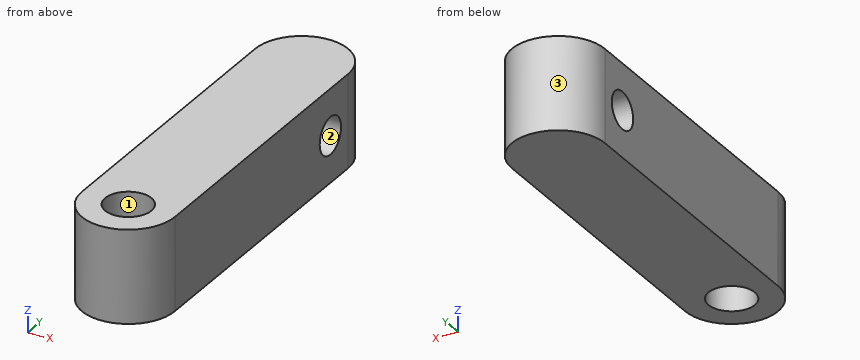
from build123d import *

# Parameters (mm, degrees)
SKETCH2_R           = 5
BOSS_EXTRUDE1_DEPTH = 20
SKETCH4_R           = 4
CUT_EXTRUDE1_DEPTH  = 55


with BuildPart() as part:
    # Sketch2 → Boss-Extrude1 (new body)
    with BuildSketch(Plane.XY):
        with BuildLine():
            Line((-10, 0), (-10, 65))
            ThreePointArc((-10, 65), (0, 75), (10, 65))
            Line((10, 65), (10, 0))
            ThreePointArc((10, 0), (0, -10), (-10, 0))
        make_face()
        Circle(SKETCH2_R, mode=Mode.SUBTRACT)
    extrude(amount=BOSS_EXTRUDE1_DEPTH)

    # Sketch4 → Cut-Extrude1 (cut)
    with BuildSketch(Plane(origin=(10, 0, 0), x_dir=(0, 0, -1), z_dir=(1, 0, 0))):
        with Locations((-10, 58.36)):
            Circle(SKETCH4_R)
    extrude(amount=-CUT_EXTRUDE1_DEPTH, mode=Mode.SUBTRACT)


solid = part.part
Verification items for the finished model (mm, model axes). Face numbers are marked on the shaded views. Round coordinates to 2 decimals unless told otherwise and drop trailing zeros. Loops run counter-clockwise (first coordinate to the right, second up) from the corner with the lowest first, then second, coordinate; pieces in that order, holes last. Notation, with made-up numbers: (17, 50.5) - (65, 50.5) arc R11 ccw to (65, 69.5) - close; hole circle Ø4 at (-38, 76). An arc over 180 degrees is marked (long way). Use a Markdown table: item, result. Add a question column.
1. Section check A-A, the plane z = 10. Record the boundary of the cut face in (x, y).
2. Section check D-D, the plane x = 7.5. Record the boundary of the cut face in (y, z), plus the area to 3 significant figures.
3. Thickness scan on probe 1 along Y at (x, z) = (0, 10); probe 2 along Y at (x, z) = (4.25, 8.75); probe 3 along Y at (x, z) = (-2.75, 19.25). Record the ranges inside material, lowest first. Write a range as [from, to].
4. Gauge pin test, flat ends, axial feed: pin 1 (3 mm diameter, centred on x = 7, z = 3, fed in from +Y); pin 2 (1 mm diameter, centred on x = 7.5, z = 7, fed in from +Y); pin 3 (1.5 mm diameter, centred on x = 5, z = 17, fed in from +Y). Record the tip position at first contact, or that the pin passes through.
5. Section check C-C, the plane y = 58.36. Record the boundary of the cut face in (x, z).
6. Release check for a two-part mould opening along X. For the marked faces 1, 2 and 3 record: released by +X, released by -X, zero draft, split by the parting line, or undercut.
7. Section check B-B, the plane x = -1. Record the boundary of the cut face in (y, z).
Checks:
| question | item | result |
|---|---|---|
| 1 | outline | (-10, 0) arc R10 ccw to (10, 0) - (10, 54.36) - (-10, 54.36) - close; (-10, 62.36) - (10, 62.36) - (10, 65) arc R10 ccw to (-10, 65) - close; hole circle Ø10 at (0, 0) |
| 2 | outline | (-6.61, 0) - (71.61, 0) - (71.61, 20) - (-6.61, 20) - close; hole circle Ø8 at (58.36, 10) |
| 2 | area | 1,510 mm^2 |
| 3 | probe 1 | y = [-10, -5], [5, 54.36], [62.36, 75] |
| 3 | probe 2 | y = [-9.05, -2.63], [2.63, 54.56], [62.16, 74.05] |
| 3 | probe 3 | y = [-9.61, -4.18], [4.18, 74.61] |
| 4 | pin 1 | stops at y = 73.35 |
| 4 | pin 2 | stops at y = 72.14 |
| 4 | pin 3 | stops at y = 74.05 |
| 5 | outline | (-10, 0) - (10, 0) - (10, 6) - (-10, 6) - close; (-10, 14) - (10, 14) - (10, 20) - (-10, 20) - close |
| 6 | face 1 | undercut |
| 6 | face 2 | zero draft |
| 6 | face 3 | split by the parting line |
| 7 | outline | (-9.95, 0) - (-4.9, 0) - (-4.9, 20) - (-9.95, 20) - close; (4.9, 0) - (74.95, 0) - (74.95, 20) - (4.9, 20) - close; hole circle Ø8 at (58.36, 10) |
